The drawing under review shows one solid part. Ordinate dimensions are in mm from its lowest x, y, z. Coordinates: 2 decimals unless noted, no trailing zeros. Loops run counter-clockwise (first coordinate to the right, second up) from the corner with the lowest first, then second, coordinate; pieces in that order, holes last. Notation, with made-up numbers: M 39,25 L 48,25 A22 ccw 48,53 Z; hole C 70,75 d11. An arc over 180 degrees is marked long. Answer as CSV lines item,"result". Start each with the question number.
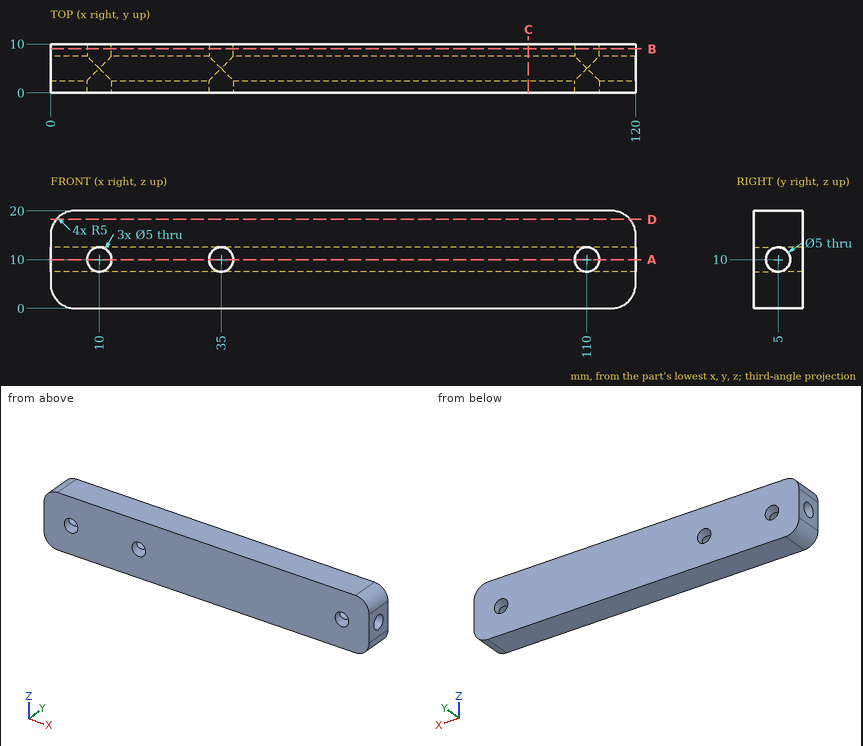
Item 1: Add section B-B (y = 9). Give the boundary of the cut face in (x, z).
Item 2: Add section A-A (z = 10). Give the number of separate pieces and of enclosed holes in the cut face, plus the area to 3 significant figures.
Item 3: Add section C-C (x = 98). Give the boundary of the cut face in (y, z).
Item 4: For line 1 along Z through (x, y) = (110, 2.75); line 2 along X through (y, z) = (9.75, 8.25); line 3 along X through (y, z) = (0.5, 9), list the stretches that pass through material, from the lowest coordinate up. Write a range as from..to.
Item 5: Add section D-D (z = 18.25). Give the boundary of the cut face in (x, y).
Response:
1,outline,"M 0,5 A5 ccw 5,0 L 115,0 A5 ccw 120,5 L 120,15 A5 ccw 115,20 L 5,20 A5 ccw 0,15 Z; hole C 10,10 d5; hole C 35,10 d5; hole C 110,10 d5"
2,separate pieces,"8"
2,enclosed holes,"0"
2,area,"525 mm²"
3,outline,"M 0,0 L 10,0 L 10,20 L 0,20 Z; hole C 5,10 d5"
4,line 1,"0..7.5, 12.5..20"
4,line 2,"0..8.21, 11.79..33.21, 36.79..108.21, 111.79..120"
4,line 3,"0..7.71, 12.29..32.71, 37.29..107.71, 112.29..120"
5,outline,"M 1.2,0 L 118.8,0 L 118.8,10 L 1.2,10 Z"
